from build123d import *

# Parameters (mm, degrees)
BOSS_EXTRUDE1_DEPTH                                  = 50.8
CBORE_FOR_1_4_BINDING_HEAD_MACHINE_SCREW_D           = 6.7564
CBORE_FOR_1_4_BINDING_HEAD_MACHINE_SCREW_CBORE_D     = 14.2875
CBORE_FOR_1_4_BINDING_HEAD_MACHINE_SCREW_CBORE_DEPTH = 3.302
SPHERICAL_HOLES_REACH                                = 75.171
SKETCH3_R                                            = 4.7625
SKETCH4_OUTSIDE_W                                    = 58.65
SKETCH4_OUTSIDE_H                                    = 67.434
ROUNDING_DEPTH                                       = 31.75


with BuildPart() as part:
    # Sketch1 → Boss-Extrude1 (new body)
    with BuildSketch(Plane.XY):
        Polygon((0, 0), (42.015665571, 0), (42.015665571, 5.5499), (8.89, 5.5499), (8.89, 26.2001), (42.015665571, 26.2001), (42.015665571, 31.75), (0, 31.75), align=None)
    extrude(amount=BOSS_EXTRUDE1_DEPTH)

    # CBORE for 1/4 Binding Head Machine Screw1 (through all)
    with Locations(Plane(origin=(8.89, 0, 0), x_dir=(0, 0, -1), z_dir=(1, 0, 0))):
        with Locations((-38.1, 15.875), (-12.7, 15.875)):
            CounterBoreHole(CBORE_FOR_1_4_BINDING_HEAD_MACHINE_SCREW_D / 2, CBORE_FOR_1_4_BINDING_HEAD_MACHINE_SCREW_CBORE_D / 2, CBORE_FOR_1_4_BINDING_HEAD_MACHINE_SCREW_CBORE_DEPTH)

    # Spherical Holes: up to this face of the body (flat: up to its plane)
    spherical_holes_end = Plane(part.part.faces().sort_by_distance((21.007832786, 31.75, 25.4))[0])
    # Sketch3 → Spherical Holes (cut, up to the picked face)
    with BuildSketch(Plane.XZ, mode=Mode.PRIVATE) as spherical_holes_sk1:
        with Locations(Location((29.315665571, 25.4, 0), (0, 0, 270))):
            Circle(SKETCH3_R)
    spherical_holes_tool1 = split(extrude(spherical_holes_sk1.sketch, amount=-SPHERICAL_HOLES_REACH, mode=Mode.PRIVATE), bisect_by=spherical_holes_end, keep=Keep.BOTH, mode=Mode.PRIVATE)
    add(spherical_holes_tool1.solids().sort_by(Axis((29.315666, 0, 25.4), (0, 1, 0)))[0], mode=Mode.SUBTRACT)

    # Sketch4 outside → Rounding (cut)
    with BuildSketch(Plane(origin=(0, 31.75, 0), x_dir=(1, 0, 0), z_dir=(0, 1, 0))):
        with Locations((21.008, -25.4)):
            Rectangle(SKETCH4_OUTSIDE_W, SKETCH4_OUTSIDE_H)
        with BuildLine():
            Line((0, 0), (34.030957579, -13.607798285))
            ThreePointArc((34.030957579, -13.607798285), (42.015665571, -25.4), (34.030957579, -37.192201715))
            Line((34.030957579, -37.192201715), (0, -50.8))
            Line((0, -50.8), (0, 0))
        make_face(mode=Mode.SUBTRACT)
    extrude(amount=-ROUNDING_DEPTH, mode=Mode.SUBTRACT)


solid = part.part
Geometry check sheet. Reference: the model listing, model coordinates, mm. A direction names the side the tool comes from. Give positions to 0.01 mm unless a question says otherwise; leave off trailing zeros. Order: outer loops, then holes, each group sorted by start corner. A loop starts at its lowest first (then second) coordinate and runs counter-clockwise, first axis right, second up.
1) Draft check along Y on faces 1 (the flat face through (5.91, 16.097, 48.437)), 2 (the flat face through (16, 0, 25)), 3 (the flat face through (5.588, 17.6, 9.6)). Enter one of: released by +Y, released by -Y, zero draft, split by the parting line, or undercut.
Results are:
face 1: zero draft
face 2: released by -Y
face 3: undercut
2) Cross-section at C-C (z = 25.4). Record the boundary of the cut face in (x, y), then the cut area to 3 significant figures.
Results are:
outline: (0, 0) - (24.55, 0) - (24.55, 5.55) - (8.89, 5.55) - (8.89, 26.2) - (24.55, 26.2) - (24.55, 31.75) - (0, 31.75) - close; (34.08, 0) - (42.02, 0) - (42.02, 5.55) - (34.08, 5.55) - close; (34.08, 26.2) - (42.02, 26.2) - (42.02, 31.75) - (34.08, 31.75) - close
area: 544 mm2
3) Cross-section at D-D (y = 17). Record the boundary of the cut face in (x, z).
Results are:
outline: (0, 0) - (8.89, 3.55) - (8.89, 5.65) - (5.59, 5.65) - (5.59, 9.51) - (0, 9.51) - close; (0, 15.89) - (5.59, 15.89) - (5.59, 19.75) - (8.89, 19.75) - (8.89, 31.05) - (5.59, 31.05) - (5.59, 34.91) - (0, 34.91) - close; (0, 41.29) - (5.59, 41.29) - (5.59, 45.15) - (8.89, 45.15) - (8.89, 47.25) - (0, 50.8) - close
4) Cross-section at A-A (z = 12.7). Record the boundary of the cut face in (x, y), then the cut area to 3 significant figures.
Results are:
outline: (0, 0) - (31.76, 0) - (31.76, 5.55) - (8.89, 5.55) - (8.89, 8.73) - (5.59, 8.73) - (5.59, 12.5) - (0, 12.5) - close; (0, 19.25) - (5.59, 19.25) - (5.59, 23.02) - (8.89, 23.02) - (8.89, 26.2) - (31.76, 26.2) - (31.76, 31.75) - (0, 31.75) - close
area: 451 mm2
5) Tool access check on faces 4 (the flat face through (5.588, 14, 35)), 5 (the flat face through (22, 26.2, 25)), 6 (the flat face through (5, 16, 2)). Record the directions out of +Z, -Z, +X, -X, +Y, -Y that give a thin tool (end or side, any length) a straight path to the whole face; none if there is none.
Results are:
face 4: +X
face 5: +Z, -Z, +X
face 6: -Z, +X, +Y, -Y
6) Material ranges on probe 1 along Y at (x, z) = (6.7, 38.1); probe 2 along Y at (x, z) = (19, 10); probe 3 along Z at (x, y) = (7, 21.5), recorded low to high.
Results are:
probe 1: y = 0 to 8.73, 23.02 to 31.75
probe 2: y = 0 to 5.55, 26.2 to 31.75
probe 3: z = 2.8 to 8.3, 17.1 to 33.7, 42.5 to 48
7) Gauge pin test, flat ends, axial feed: pin 1 (12 mm diameter, centred on y = 19, z = 24.5, fed in from +X); pin 2 (3 mm diameter, centred on x = 8.5, y = 8, fed in from +Z); pin 3 (10 mm diameter, centred on y = 14, z = 26.5, fed in from -X); pin 4 (6 mm diameter, centred on x = 17, y = 25.5, fed in from -Z). Record the tip position at first contact, or that the pin passes through.
Results are:
pin 1: stops at x = 8.89
pin 2: stops at z = 48
pin 3: stops at x = 0
pin 4: stops at z = 5.63
8) Cross-section at B-B (x = 31). Record the boundary of the cut face in (y, z), then the cut area to 3 significant figures.
Results are:
outline: (0, 12.4) - (5.55, 12.4) - (5.55, 20.95) - (0, 20.95) - close; (0, 29.85) - (5.55, 29.85) - (5.55, 38.4) - (0, 38.4) - close; (26.2, 12.4) - (31.75, 12.4) - (31.75, 20.95) - (26.2, 20.95) - close; (26.2, 29.85) - (31.75, 29.85) - (31.75, 38.4) - (26.2, 38.4) - close
area: 190 mm2
